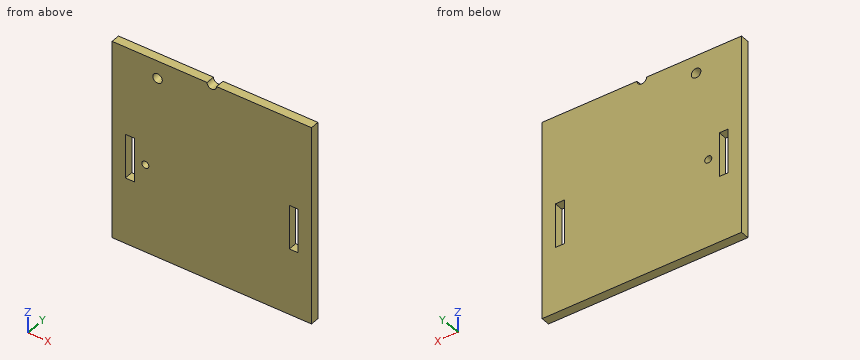
Autodesk Fusion 360 part; units mm, degrees
sketch "スケッチ1" plane through (0, 0, 0) normal (0, 1, 0) x (1, 0, 0)
  line L0 (-45, 0) -> (45, 0)
  line L1 (45, 0) -> (45, 90)
  line L2 (45, 90) -> (-45, 90)
  line L3 (-45, 90) -> (-45, 0)
  line L4 (-39, 60) -> (-35, 60)
  line L5 (-35, 60) -> (-35, 40)
  line L6 (-35, 40) -> (-39, 40)
  line L7 (-39, 40) -> (-39, 60)
  line L8 (35, 60) -> (39, 60)
  line L9 (39, 60) -> (39, 40)
  line L10 (39, 40) -> (35, 40)
  line L11 (35, 40) -> (35, 60)
  line L12 (-24.5, 83) -> (24.5, 83)
  line L13 (24.5, 83) -> (24.5, 8)
  line L14 (24.5, 8) -> (-24.5, 8)
  line L15 (-24.5, 8) -> (-24.5, 83)
  line L16 (-35, 50) -> (-30, 50)
  line L17 (35, 50) -> (30, 50)
  point P0 (0, 8)
  dimension "d1" = 90
  dimension "d2" = 90
  dimension "d3" = 40
  dimension "d4" = 20
  dimension "d5" = 4
  dimension "d6" = 35
  dimension "d7" = 35
  dimension "d8" = 49
  dimension "d9" = 75
  dimension "d10" = 8
  dimension "d16" = 5
  dimension "d17" = 5
extrude "押し出し1" add sketch "スケッチ1" along normal blind 4 contours L0 L1 L2 L3 | L12 L13 L14 L15
hole "穴1" at (-24.5, 0, -8) at (0, 0, 0) at (0, 0, 0) at (0, 0, 0) direction (0, 1, 0) diameter 4.3 depth 4 tip angle 118
hole "穴2" at (-30, 0, -50) at (0, 0, 0) direction (0, 1, 0) diameter 3.2 end through all
Here's how the part is built. I have some questions about the finished solid (model axes, mm). Coordinates: 2 decimals unless noted, no trailing zeros. Loops run counter-clockwise (first coordinate to the right, second up) from the corner with the lowest first, then second, coordinate; pieces in that order, holes last. Notation, with made-up numbers: M 80,7.5 L 120,7.5 A20 cw 120,32.5 Z; hole C -18,26 d11. An arc over 180 degrees is marked long. One line per item, written item: value.
1. Imagine slicing it at B-B (y = 1.1). List the corners of the cut face in (x, z) for me, and give its area (3 significant figures).
Geometry says:
outline: M -45,-90 L 45,-90 L 45,0 L 2.15,0 A2.15 cw -2.15,0 L -45,0 Z; hole M -39,-60 L -35,-60 L -35,-40 L -39,-40 Z; hole C -30,-50 d3.2; hole C -24.5,-8 d4.3; hole M 35,-60 L 39,-60 L 39,-40 L 35,-40 Z
area: 7,910 mm2
2. Please list where these lines run through material, in increasing order: probe 1 along X at (y, z) = (1.35, -50); probe 2 along X at (y, z) = (2.05, -45); probe 3 along Z at (x, y) = (-24.5, 2.7).
Geometry says:
probe 1: x = -45 to -39, -35 to -31.6, -28.4 to 35, 39 to 45
probe 2: x = -45 to -39, -35 to 35, 39 to 45
probe 3: z = -90 to -10.15, -5.85 to 0
3. Imagine slicing it at C-C (z = -56). List the corners of the cut face in (x, y) for me, and give its area (3 significant figures).
Geometry says:
outline: M -45,0 L -39,0 L -39,4 L -45,4 Z; M -35,0 L 35,0 L 35,4 L -35,4 Z; M 39,0 L 45,0 L 45,4 L 39,4 Z
area: 328 mm2
4. Imagine slicing it at A-A (x = -30). List the corners of the cut face in (y, z) for me.
Geometry says:
outline: M 0,-90 L 4,-90 L 4,-51.6 L 0,-51.6 Z; M 0,-48.4 L 4,-48.4 L 4,0 L 0,0 Z
5. Imagine slicing it at D-D (x = 0). List the corners of the cut face in (y, z) for me.
Geometry says:
outline: M 0,-90 L 4,-90 L 4,-2.15 L 0,-2.15 Z
